Job drawing, mm, ordinate dimensions from the low corner. One solid piece. A direction names the side the tool comes from. Give positions to 0.01 mm unless a question says otherwise; leave off trailing zeros. Loops run counter-clockwise (first coordinate to the right, second up) from the corner with the lowest first, then second, coordinate; pieces in that order, holes last.
Item 1: Probe probe 1 along Z at (x, y) = (20, 0.8) (1 decimal); probe 2 along X at (y, z) = (6, 3.75); probe 3 along Z at (x, y) = (35, 5.6) (1 decimal). List the from-to ranges inside material, lowest first.
Item 2: Saw through at C-C on y = 2.25. Give the cut face in (x, z) (1 decimal).
Item 3: Saw through at A-A on z = 15.75. Give the cut face in (x, y).
Item 4: Saw through at B-B on x = 5. Give the cut face in (y, z) (1 decimal).
Item 5: Drop flat-ended pins along their axis: P1, Ø3.5, axis at x = 5.5, z = 9, coming from the -Y side; P2, Ø2.5, axis at x = 20, z = 8.445, coming from the -Y side; P3, Ø8, axis at x = 35, z = 7.5, coming from the -Y side; P4, Ø1.8, axis at y = 2, z = 8.5, coming from the -X side. Give the stop position or say it passes through.
Item 6: Mould opens along X. For the marked faces 6, 7, 8 and 9 say: released by +X, released by -X, zero draft, split by the parting line, or undercut.
Item 7: Which spindle directions (+Z, -Z, +X, -X, +Y, -Y) get a long thin tool onto all of the face, cutting with end or side? Do the marked faces 1, 2, 3, 4 and 5. Say none if no direction does.
Item 8: Saw through at D-D on x = 20. Give the cut face in (y, z) (1 decimal).
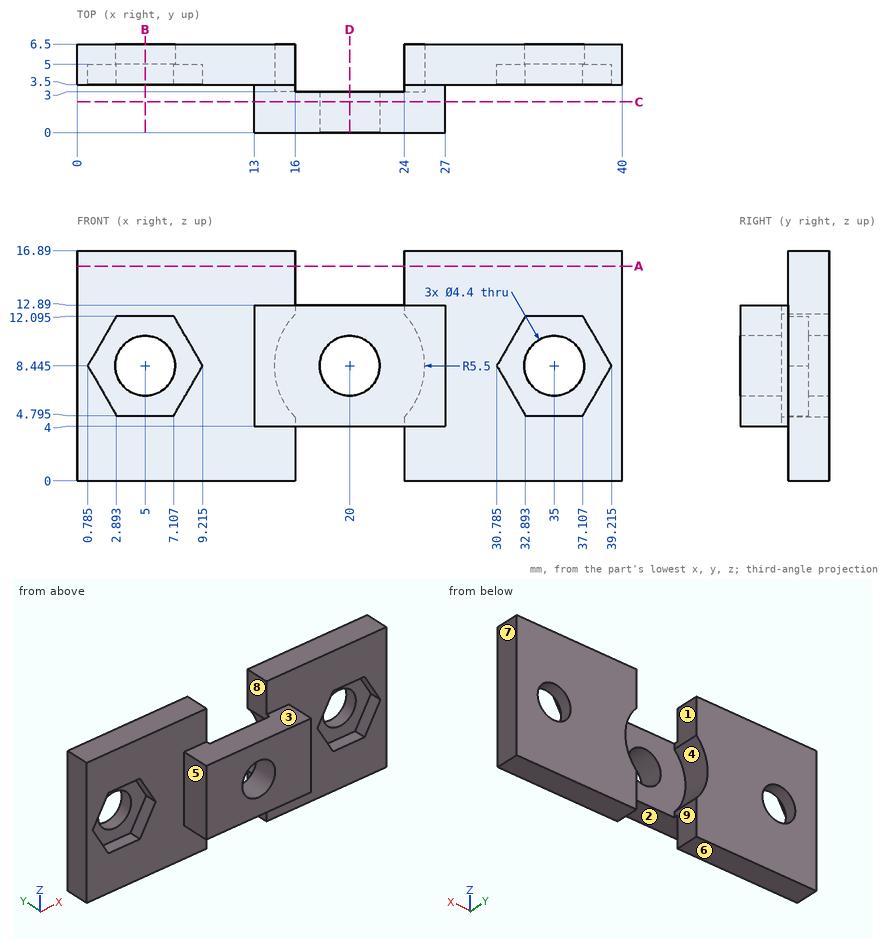
Results below:
1. probe 1: z = 4 to 6.2, 10.6 to 12.9
1. probe 2: x = 0 to 16, 24 to 40
1. probe 3: z = 0 to 6.2, 10.6 to 16.9
2. outline: (13, 4) - (27, 4) - (27, 12.9) - (13, 12.9) - close; hole circle Ø4.4 at (20, 8.4)
3. outline: (0, 3.5) - (16, 3.5) - (16, 6.5) - (0, 6.5) - close; (24, 3.5) - (40, 3.5) - (40, 6.5) - (24, 6.5) - close
4. outline: (3.5, 0) - (6.5, 0) - (6.5, 6.2) - (5, 6.2) - (5, 4.8) - (3.5, 4.8) - close; (3.5, 12.1) - (5, 12.1) - (5, 10.6) - (6.5, 10.6) - (6.5, 16.9) - (3.5, 16.9) - close
5. P1: stops at y = 5
5. P2: passes through
5. P3: stops at y = 3.5
5. P4: stops at x = 13
6. face 6: zero draft
6. face 7: released by +X
6. face 8: undercut
6. face 9: undercut
7. face 1: +Z, -Z, +Y
7. face 2: -Z, +X, -X, -Y
7. face 3: +Z, +X, -X, -Y
7. face 4: +Y
7. face 5: +Z, -Z, -X, -Y
8. outline: (0, 4) - (3, 4) - (3, 6.2) - (0, 6.2) - close; (0, 10.6) - (3, 10.6) - (3, 12.9) - (0, 12.9) - close
